Verification items for the finished model (mm, model axes). A direction names the side the tool comes from. Coordinates: 2 decimals unless noted, no trailing zeros. Write each loop counter-clockwise with the first axis right and the second up, starting at its lowest first coordinate (ties: lowest second). Pieces come first, ordered by that corner, then holes. Notation, with made-up numbers: (7.25, 89.5) -> (46.25, 89.5) arc R6 ccw to (46.25, 93.5) -> close; hole circle Ø10 at (67, -25.5). An arc over 180 degrees is marked (long way). Use a Markdown table: item, result. Add a question column.
from build123d import *

# Parameters (mm, degrees)
SKETCH_1_W                   = 60
SKETCH_1_H                   = 25
EXTRUDE_1_DEPTH              = 8
EXTRUDE_2_DEPTH              = 6
EXTRUDE_2_DEPTH_BACK         = 8
SKETCH_2_W                   = 60
SKETCH_2_H                   = 8
CUT_EXTRUDE_1_DEPTH          = 65.932657423
CUT_EXTRUDE_1_DEPTH_BACK     = 65.932657423
SKETCH_3_W                   = 6
SKETCH_3_H                   = 0.8
HOLE_WIZARD_M4_1_D           = 4.8
HOLE_WIZARD_M4_1_DEPTH       = 10.1
HOLE_WIZARD_M4_1_CBORE_D     = 8
HOLE_WIZARD_M4_1_CBORE_DEPTH = 4
HOLE_WIZARD_M4_1_TIP         = 1.442065486
SKETCH_7_W                   = 14
SKETCH_7_H                   = 7.2
EXTRUDE_3_DEPTH              = 50


with BuildPart() as part:
    # 스케치1 → 보스-돌출1 (new body)
    with BuildSketch(Plane.XY):
        Rectangle(SKETCH_1_W, SKETCH_1_H)
    extrude(amount=EXTRUDE_1_DEPTH)

    # 스케치2 → 보스-돌출2 (add, two sides: drawn at the far end of the back side and taken through both)
    with BuildSketch(Plane.XY.offset(8).offset(-EXTRUDE_2_DEPTH_BACK)):
        with Locations((0, 16.5)):
            Rectangle(SKETCH_2_W, SKETCH_2_H)
    extrude(amount=EXTRUDE_2_DEPTH + EXTRUDE_2_DEPTH_BACK)

    # 스케치3 → 컷-돌출1 (cut, two sides: drawn at the far end of the back side and taken through both)
    with BuildSketch(Plane(origin=(30, 0, 0), x_dir=(0, 0, -1), z_dir=(1, 0, 0)).offset(-CUT_EXTRUDE_1_DEPTH_BACK)):
        with Locations((-11, 12.9)):
            Rectangle(SKETCH_3_W, SKETCH_3_H)
    extrude(amount=CUT_EXTRUDE_1_DEPTH + CUT_EXTRUDE_1_DEPTH_BACK, mode=Mode.SUBTRACT)

    # M4 소켓 머리 캡 나사용 카운터보어1
    with Locations(Plane(origin=(0, 0, 0), x_dir=(-1, 0, 0), z_dir=(0, 0, -1))):
        with Locations((-20, -2.5), (20, -2.5)):
            CounterBoreHole(HOLE_WIZARD_M4_1_D / 2, HOLE_WIZARD_M4_1_CBORE_D / 2, HOLE_WIZARD_M4_1_CBORE_DEPTH, depth=HOLE_WIZARD_M4_1_DEPTH)
            with Locations((0, 0, -(HOLE_WIZARD_M4_1_DEPTH + HOLE_WIZARD_M4_1_TIP / 2))):  # 118° drill point
                Cone(0, HOLE_WIZARD_M4_1_D / 2, HOLE_WIZARD_M4_1_TIP, mode=Mode.SUBTRACT)

    # 스케치7 → 보스-돌출3 (add)
    with BuildSketch(Plane.ZY.offset(-30)):
        with Locations((7, 16.9)):
            Rectangle(SKETCH_7_W, SKETCH_7_H)
    extrude(amount=-EXTRUDE_3_DEPTH)


solid = part.part
1) Cross-section at B-B on x = -20. Record the boundary of the cut face in (y, z).
2) Set-up check for faces 1 (the face through (80, 17, 7)), 2 (the face through (0, 1, 8)), 3 (the face through (23.2, -4.9, 2)): record each of +Z, -Z, +X, -X, +Y, -Y from which the full face is reachable in a straight line by a thin tool's end or side.
3) Cross-section at C-C on z = 6.75. Record the boundary of the cut face in (x, y), then the cut area to 3 significant figures.
4) Thickness scan on L1, parallel to Y at x = 20, z = 5.4; L2, parallel to Y at x = 20, z = 2.75; L3, parallel to X at y = -4, z = 7. Record the ranges inside material, lowest first.
5) Cross-section at A-A on y = -2.5. Record the boundary of the cut face in (x, z), then the cut area to 3 significant figures.
6) Cross-section at D-D on y = 11.5. Record the boundary of the cut face in (x, z), then the cut area to 3 significant figures.
7) Release check for a two-part mould opening along Y. For faces 4 (the face through (-17.71, -1.78, 6.03)), 5 (the face through (0, -12.5, 4)), 6 (the face through (30, 0, 4)) record: released by +Y, released by -Y, zero draft, split by the parting line, or undercut.
8) Gauge pin test, flat ends, axial feed: pin 1 (10 mm diameter, centred on x = 25, y = 9.5, fed in from +Z); pin 2 (4 mm diameter, centred on y = -5.5, z = 2.5, fed in from +X); pin 3 (4.5 mm diameter, centred on x = 20, y = -2.5, fed in from -Z); pin 4 (7 mm diameter, centred on x = 35, z = 7.5, fed in from -Y). Record the tip position at first contact, or that the pin passes through.
Returned:
| question | item | result |
|---|---|---|
| 1 | outline | (-12.5, 0) -> (-6.5, 0) -> (-6.5, 4) -> (-4.9, 4) -> (-4.9, 8) -> (-12.5, 8) -> close; (-0.1, 4) -> (1.5, 4) -> (1.5, 0) -> (20.5, 0) -> (20.5, 14) -> (13.3, 14) -> (13.3, 8) -> (-0.1, 8) -> close |
| 2 | face 1 | +Z, -Z, +X, +Y, -Y |
| 2 | face 2 | +Z, +X, -X, -Y |
| 2 | face 3 | -Z |
| 3 | outline | (-30, -12.5) -> (30, -12.5) -> (30, 13.3) -> (80, 13.3) -> (80, 20.5) -> (-30, 20.5) -> close; hole circle Ø4.8 at (-20, -2.5); hole circle Ø4.8 at (20, -2.5) |
| 3 | area | 2,300 mm² |
| 4 | L1 | y = -12.5 to -4.9, -0.1 to 20.5 |
| 4 | L2 | y = -12.5 to -6.5, 1.5 to 20.5 |
| 4 | L3 | x = -30 to -21.87, -18.13 to 18.13, 21.87 to 30 |
| 5 | outline | (-30, 0) -> (-24, 0) -> (-24, 4) -> (-22.4, 4) -> (-22.4, 8) -> (-30, 8) -> close; (-17.6, 4) -> (-16, 4) -> (-16, 0) -> (16, 0) -> (16, 4) -> (17.6, 4) -> (17.6, 8) -> (-17.6, 8) -> close; (22.4, 4) -> (24, 4) -> (24, 0) -> (30, 0) -> (30, 8) -> (22.4, 8) -> close |
| 5 | area | 378 mm² |
| 6 | outline | (-30, 0) -> (30, 0) -> (30, 8) -> (-30, 8) -> close |
| 6 | area | 480 mm² |
| 7 | face 4 | undercut |
| 7 | face 5 | released by -Y |
| 7 | face 6 | zero draft |
| 8 | pin 1 | stops at z = 14 |
| 8 | pin 2 | stops at x = 30 |
| 8 | pin 3 | passes through |
| 8 | pin 4 | stops at y = 13.3 |
